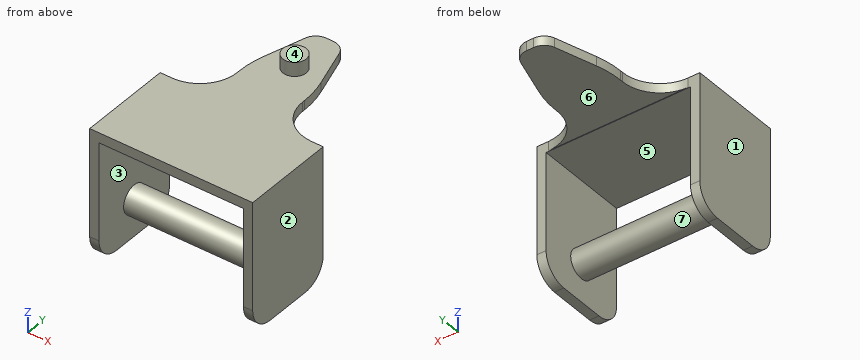
Solid Edge part; units mm, degrees
sketch "Sketch1" plane through (0, 0, 0) normal (1, 0, 0) x (0, 1, 0)
  circle A0 centre (0, 0) radius 3.025
extrude "Protrusion1" add sketch "Sketch1" along normal mid plane 31
sketch "Sketch2" plane through (0, 0, 0) normal (0, -1, 0) x (1, 0, 0)
  line L0 (15.5, 18) -> (15.5, 0)
  line L1 (15.5, 0) -> (15.5, -8)
  line L2 (15.5, -8) -> (17.5, -8)
  line L3 (17.5, -8) -> (17.5, 18)
  line L4 (17.5, 18) -> (17.5, 20.1428)
  line L5 (-17.5, 20.1428) -> (17.5, 20.1428)
  line L6 (-17.5, 18) -> (-17.5, 20.1428)
  line L7 (-17.5, -8) -> (-17.5, 18)
  line L8 (-15.5, -8) -> (-17.5, -8)
  line L9 (-15.5, 0) -> (-15.5, -8)
  line L10 (-15.5, 18) -> (-15.5, 0)
  line L11 (-15.5, 18) -> (15.5, 18)
  dimension "D1" = 15.5
extrude "ExtrudedProtrusion_2" add sketch "Sketch2" along normal mid plane 20
fillet "Round_1" radius 5 4 edges at (16.5, 10, -8) (-16.5, 10, -8) (-16.5, -10, -8) (16.5, -10, -8)
sketch "Sketch3" plane through (0, 0, 20.1428) normal (0, 0, 1) x (0, -1, 0)
  line L0 (-18.5994, 7) -> (-18, 7)
  arc A0 (-10, 15) -> (-18, 7) centre (-18, 15) cw
  line L1 (-10, 15) -> (-10, 17.5)
  line L2 (-10, 17.5) -> (-6.9702, 17.5)
  line L3 (-6.9702, 17.5) -> (-6.9702, -17.5)
  line L4 (-6.9702, -17.5) -> (-10, -17.5)
  line L5 (-10, -15) -> (-10, -17.5)
  arc A1 (-18, -7) -> (-10, -15) centre (-18, -15) cw
  line L6 (-18.5994, -7) -> (-18, -7)
  arc A2 (-24.2811, -6.176) -> (-18.5994, -7) centre (-18.5994, 13) ccw
  line L7 (-32.8523, -3.6364) -> (-24.2811, -6.176)
  arc A3 (-35, -0.76) -> (-32.8523, -3.6364) centre (-32, -0.76) ccw
  line L8 (-35, 0) -> (-35, -0.76)
  line L9 (-35, 0) -> (-35, 0.76)
  arc A4 (-32.8523, 3.6364) -> (-35, 0.76) centre (-32, 0.76) ccw
  line L10 (-32.8523, 3.6364) -> (-24.2811, 6.176)
  arc A5 (-24.2811, 6.176) -> (-18.5994, 7) centre (-18.5994, -13) cw
extrude "ExtrudedProtrusion_3" add sketch "Sketch3" against normal blind 2
sketch "Sketch4" plane through (0, 12.5, 20.1428) normal (0, 0, 1) x (0, -1, 0)
  circle A0 centre (-12.5, 0) radius 2.5
extrude "Protrusion2" add sketch "Sketch4" along normal up to vertex (3 mm away)
properties material "Steel, structural"
Input: part model. Units: mm. Frame: model coordinates. Face numbers are marked on the shaded views. A direction names the side the tool comes from. Give positions to 0.01 mm unless a question says otherwise; leave off trailing zeros. Order: outer loops, then holes, each group sorted by start corner. A loop starts at its lowest first (then second) coordinate and runs counter-clockwise, first axis right, second up.
Q1. Set-up query: the marked faces 5, 6 and 7. Return all of +Z, -Z, +X, -X, +Y, -Y with unobstructed straight access to the full face (end or side cutting, diameter ignored); none if empty.
Checked values:
face 5: +Y, -Y
face 6: -Z, +X, -X, +Y
face 7: none
Q2. Contact query for flat-ended pins moving along their axis: pin 1 Ø1.5 at (x, y) = (1.5, 5.5) entering from +Z; pin 2 Ø0.5 at (y, z) = (18, 18.5) entering from +X; pin 3 Ø3 at (x, z) = (13, -2) entering from +Y. Output: stop coordinate, or through.
Checked values:
pin 1: stops at z = 20.14
pin 2: stops at x = 7
pin 3: stops at y = 2.98
Q3. Draft query along X for the marked faces 1, 2, 3 and 4. Return one class per face: +X half, -X half, draft (parallel to the pull), parting line (faces both ways), or undercut.
Checked values:
face 1: -X half
face 2: +X half
face 3: undercut
face 4: draft
Q4. Section A-A on y = 0. Output: boundary loops of the cut face in (x, z) (3 decimals).
Checked values:
outline: (-17.5, -8) - (-15.5, -8) - (-15.5, -3.025) - (15.5, -3.025) - (15.5, -8) - (17.5, -8) - (17.5, 20.143) - (-17.5, 20.143) - close; hole (-15.5, 3.025) - (15.5, 3.025) - (15.5, 18) - (-15.5, 18) - close
Q5. Section D-D on z = -2. Output: boundary loops of the cut face in (x, y).
Checked values:
outline: (-17.5, -10) - (-15.5, -10) - (-15.5, -2.27) - (15.5, -2.27) - (15.5, -10) - (17.5, -10) - (17.5, 10) - (15.5, 10) - (15.5, 2.27) - (-15.5, 2.27) - (-15.5, 10) - (-17.5, 10) - close
Q6. Section C-C on x = 0. Output: boundary loops of the cut face in (y, z) (3 decimals).
Checked values:
outline: (-10, 18) - (10, 18) - (10, 18.143) - (35, 18.143) - (35, 20.143) - (27.5, 20.143) - (27.5, 23.143) - (22.5, 23.143) - (22.5, 20.143) - (-10, 20.143) - close; circle Ø6.05 at (0, 0)
Q7. Ray query, probe 1 along X at (y, z) = (-3, 10); probe 2 along Z at (x, y) = (-10, 11); probe 3 along Z at (x, y) = (-8.5, 4). Return the intervals inside material, ascending.
Checked values:
probe 1: x = -17.5 to -15.5, 15.5 to 17.5
probe 2: z = 18.14 to 20.14
probe 3: z = 18 to 20.14
Q8. Section B-B on z = 13. Output: boundary loops of the cut face in (x, y), and give its area (3 significant figures).
Checked values:
outline: (-17.5, -10) - (-15.5, -10) - (-15.5, 10) - (-17.5, 10) - close; (15.5, -10) - (17.5, -10) - (17.5, 10) - (15.5, 10) - close
area: 80.0 mm2
